Verification items for this drawing (mm, ordinates from the low corner). Give positions to 0.01 mm unless a question says otherwise; leave off trailing zeros. Loops run counter-clockwise (first coordinate to the right, second up) from the corner with the lowest first, then second, coordinate; pieces in that order, holes last. Notation, with made-up numbers: (-28, 20.5) -> (18, 20.5) arc R23 ccw to (18, 54.5) -> close; hole circle Ø5 at (76.5, 52.25). An arc over 180 degrees is marked (long way). Write item = value, one per line.
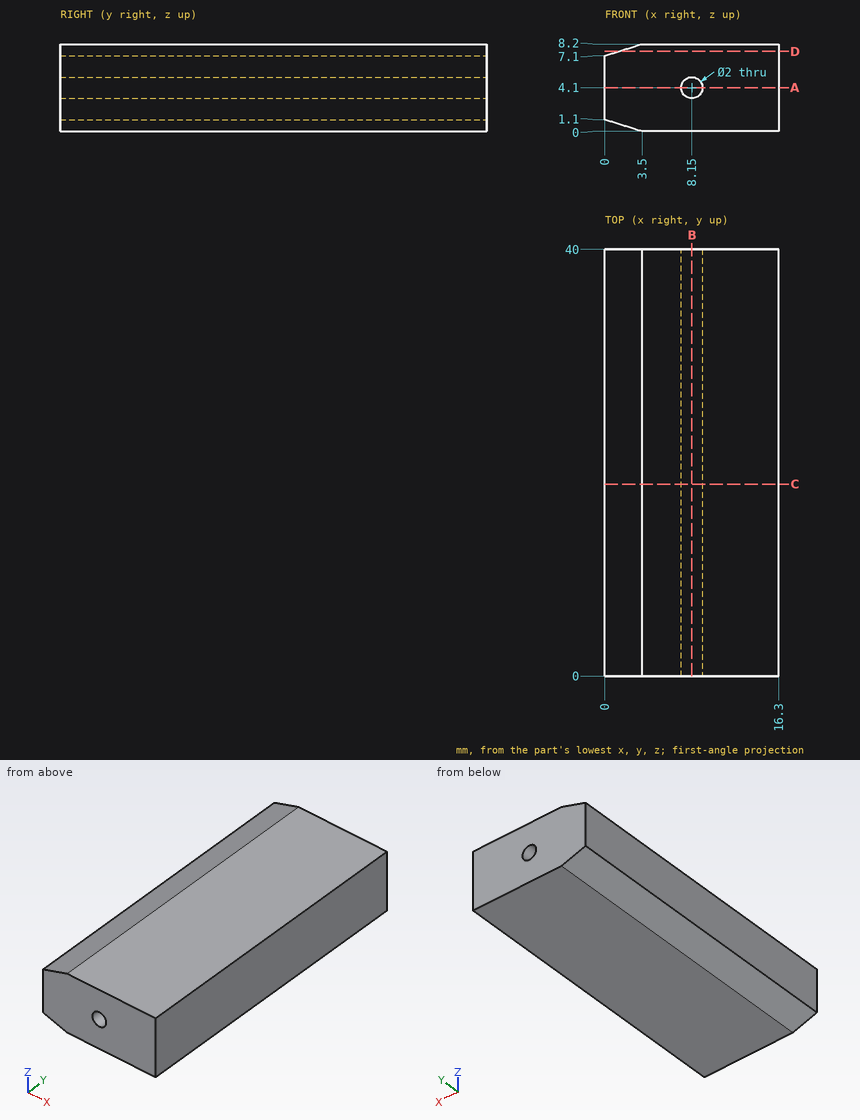
Item 1: Section check B-B, the plane x = 8.15. Record the cut outline in (y, z), plus the area to 3 significant figures.
Answer:
outline = (0, 0) -> (40, 0) -> (40, 3.1) -> (0, 3.1) -> close; (0, 5.1) -> (40, 5.1) -> (40, 8.2) -> (0, 8.2) -> close
area = 248 mm^2
Item 2: Section check D-D, the plane z = 7.5. Record the cut outline in (x, y).
Answer:
outline = (1.27, 0) -> (16.3, 0) -> (16.3, 40) -> (1.27, 40) -> close
Item 3: Thickness scan on L1, parallel to X at y = 17, z = 4.1; L2, parallel to Z at x = 8.15, y = 17.5; L3, parallel to Z at x = 7.5, y = 11. Record the ranges inside material, lowest first. Write a range as [from, to].
Answer:
L1 = [0, 7.15], [9.15, 16.3]
L2 = [0, 3.1], [5.1, 8.2]
L3 = [0, 3.34], [4.86, 8.2]
Item 4: Section check C-C, the plane y = 18. Record the cut outline in (x, z).
Answer:
outline = (0, 1.1) -> (3.5, 0) -> (16.3, 0) -> (16.3, 8.2) -> (3.5, 8.2) -> (0, 7.1) -> close; hole circle Ø2 at (8.15, 4.1)
Item 5: Section check A-A, the plane z = 4.1. Record the cut outline in (x, y), plus the area to 3 significant figures.
Answer:
outline = (0, 0) -> (7.15, 0) -> (7.15, 40) -> (0, 40) -> close; (9.15, 0) -> (16.3, 0) -> (16.3, 40) -> (9.15, 40) -> close
area = 572 mm^2
